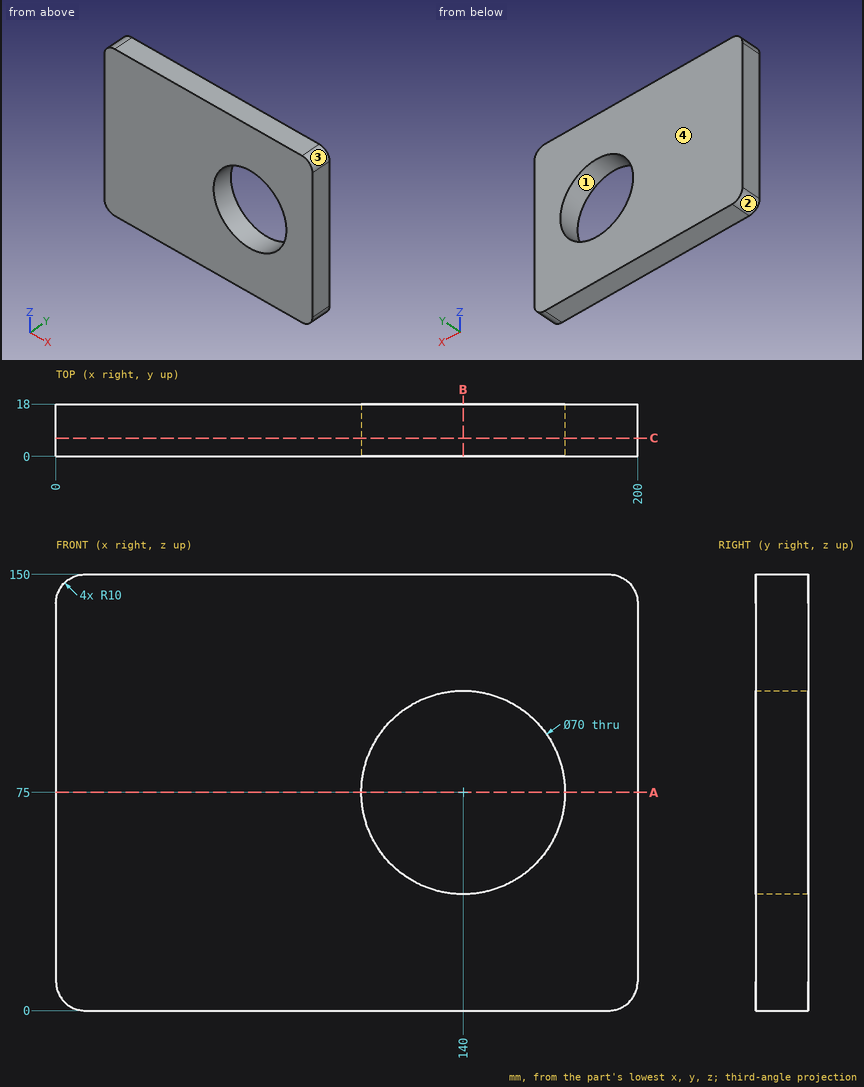
Could you check a few things on this drawing? It's one solid part, dimensions in mm from its lowest x, y, z. Round coordinates to 2 decimals unless told otherwise and drop trailing zeros. Order: outer loops, then holes, each group sorted by start corner. A loop starts at its lowest first (then second) coordinate and runs counter-clockwise, first axis right, second up.
Q1. Imagine slicing it at A-A, the plane z = 75. List the corners of the cut face in (x, y) for me.
Geometry says:
outline: (0, 0) - (105, 0) - (105, 18) - (0, 18) - close; (175, 0) - (200, 0) - (200, 18) - (175, 18) - close
Q2. Thinking about a two-plate mould opening in X: for the marked faces 1, 2, 3 and 4, which applies, released by +X, released by -X, zero draft, split by the parting line, or undercut?
Geometry says:
face 1: undercut
face 2: released by -X
face 3: released by +X
face 4: zero draft
Q3. Imagine slicing it at B-B, the plane x = 140. List the corners of the cut face in (y, z) for me.
Geometry says:
outline: (0, 0) - (18, 0) - (18, 40) - (0, 40) - close; (0, 110) - (18, 110) - (18, 150) - (0, 150) - close
Q4. Please list where these lines run through material, in increasing order: probe 1 along X at (y, z) = (14, 75); probe 2 along X at (y, z) = (14.5, 78); probe 3 along Z at (x, y) = (150, 8.25).
Geometry says:
probe 1: x = 0 to 105, 175 to 200
probe 2: x = 0 to 105.13, 174.87 to 200
probe 3: z = 0 to 41.46, 108.54 to 150
Q5. Imagine slicing it at C-C, the plane y = 6.25. List the corners of the cut face in (x, z) for me.
Geometry says:
outline: (0, 10) arc R10 ccw to (10, 0) - (190, 0) arc R10 ccw to (200, 10) - (200, 140) arc R10 ccw to (190, 150) - (10, 150) arc R10 ccw to (0, 140) - close; hole circle Ø70 at (140, 75)
